Design review of the part built by this model. Coordinates are the model's own, in mm. Face numbers are marked on the shaded views. Coordinates: 2 decimals unless noted, no trailing zeros. Write each loop counter-clockwise with the first axis right and the second up, starting at its lowest first coordinate (ties: lowest second). Pieces come first, ordered by that corner, then holes.
Q1. The part is to be moulded in two halves that separate along Y. For the marked faces 1, 2 and 3, say which applies: +Y half, -Y half, draft (parallel to the pull), parting line (faces both ways), or undercut.
Q2. To check wall thickness, follow probe 1 along Y at (x, z) = (0, 0.7); probe 2 along Z at (x, y) = (31.5, -28); probe 3 along Y at (x, z) = (-17, 12.5). State the ranges of each line that lie inside material, in increasing order.
Q3. Clearance check with flat-ended pins moving along their axes: pin 1 Ø10 at (x, z) = (6, 44) entering from -Y; pin 2 Ø10 at (x, y) = (-12, 11) entering from +Z; pin 3 Ø2.5 at (x, y) = (-46, 5.5) entering from +Z; pin 4 Ø9.5 at (x, y) = (0, 0) entering from +Z. State where each tip first meets the part, or that it passes through.
Q4. Add section A-A, the plane z = 16. Give the boundary of the cut face in (x, y), plus the area to 3 significant figures.
Q5. Add section C-C, the plane y = 40. Give the boundary of the cut face in (x, z).
Q6. Add section B-B, the plane x = 0. Give the boundary of the cut face in (y, z).
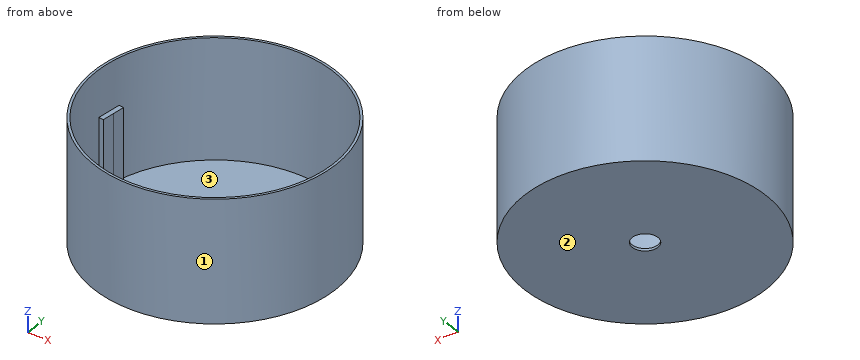
from build123d import *

# Parameters (mm, degrees)
F0_R     = 49.5
F0_R_2   = 48.5
F1_DEPTH = 50
F0_R_3   = 5.25
F2_DEPTH = 1
F4_DEPTH = 30


with BuildPart() as f1:
    # F0 (on Top) → F1 (new body)
    with BuildSketch(Plane.XY):
        Circle(F0_R)
        Circle(F0_R_2, mode=Mode.SUBTRACT)
    extrude(amount=F1_DEPTH)

    # F0 (on Top) → F2 (join)
    with BuildSketch(Plane.XY):
        Circle(F0_R_2)
        Circle(F0_R_3, mode=Mode.SUBTRACT)
    extrude(amount=F2_DEPTH)

    # F3 (on face) → F4 (join)
    with BuildSketch(Plane.XY.offset(1)):
        Polygon((-47.02107, 11.233586), (-47.673701, 6.276362), (-45.690812, 6.015309), (-45.038181, 10.972534), align=None)
        Polygon((-47.673701, 6.276362), (-48.326332, 1.319138), (-46.343443, 1.058085), (-45.690812, 6.015309), align=None)
    extrude(amount=F4_DEPTH)


solid = f1.part
Here are the results:
1. face 1: parting line
1. face 2: draft
1. face 3: undercut
2. probe 1: y = -49.5 to -5.25, 5.25 to 49.5
2. probe 2: z = 0 to 1
2. probe 3: y = -46.49 to -45.42, 45.42 to 46.49
3. pin 1: stops at y = -49.49
3. pin 2: stops at z = 1
3. pin 3: stops at z = 31
3. pin 4: passes through
4. outline: circle Ø99 at (0, 0); (-48.33, 1.32) - (-46.34, 1.06) - (-45.04, 10.97) - (-47.02, 11.23) - close; hole circle Ø97 at (0, 0)
4. area: 328 mm2
5. outline: (-29.16, 0) - (29.16, 0) - (29.16, 50) - (27.43, 50) - (27.43, 1) - (-27.43, 1) - (-27.43, 50) - (-29.16, 50) - close
6. outline: (-49.5, 0) - (-5.25, 0) - (-5.25, 1) - (-48.5, 1) - (-48.5, 50) - (-49.5, 50) - close; (5.25, 0) - (49.5, 0) - (49.5, 50) - (48.5, 50) - (48.5, 1) - (5.25, 1) - close
